```python
from build123d import *

# Parameters (mm, degrees)
SKETCH1_W           = 226
SKETCH1_H           = 170
BOSS_EXTRUDE1_DEPTH = 5
SKETCH2_W           = 226
SKETCH2_H           = 170
BOSS_EXTRUDE2_DEPTH = 4


with BuildPart() as part:
    # Sketch1 → Boss-Extrude1 (new body)
    with BuildSketch(Plane(origin=(0, 0, 0), x_dir=(1, 0, 0), z_dir=(0, 1, 0))):
        Polygon((234, -94), (234, -178), (0, -178), (0, 0), (234, 0), (234, -84), (244, -84), (244, -94), align=None)
        with Locations((117, -89)):
            Rectangle(SKETCH1_W, SKETCH1_H, mode=Mode.SUBTRACT)
    extrude(amount=BOSS_EXTRUDE1_DEPTH)

    # Sketch2 → Boss-Extrude2 (add)
    with BuildSketch(Plane(origin=(0, 0, 0), x_dir=(1, 0, 0), z_dir=(0, 1, 0))):
        with Locations((117, -89)):
            Rectangle(SKETCH2_W, SKETCH2_H)
    extrude(amount=BOSS_EXTRUDE2_DEPTH)


solid = part.part
```
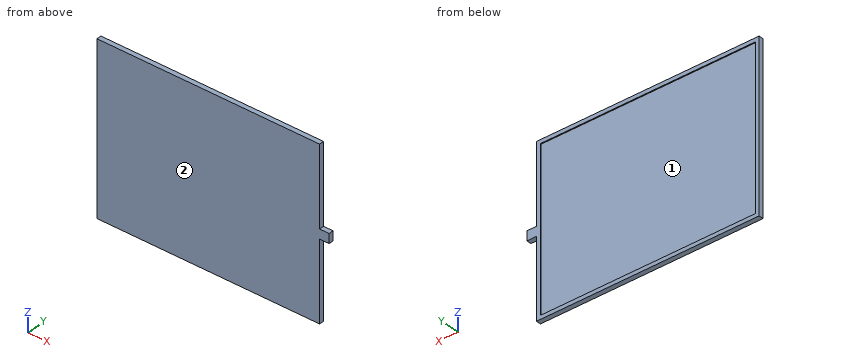
The listing builds one solid part. Answer for the finished solid, in the listing's coordinates (mm). Face numbers are marked on the shaded views. Give positions to 0.01 mm unless a question says otherwise; leave off trailing zeros. Order: outer loops, then holes, each group sorted by start corner. A loop starts at its lowest first (then second) coordinate and runs counter-clockwise, first axis right, second up. Notation, with made-up numbers: (53, 23) -> (62, 23) arc R21 cw to (62, 58) -> close; hole circle Ø5 at (70.5, 36). An arc over 180 degrees is marked (long way). Answer as a JSON object with one key per item and string values. Group by question number.
Item 1: Consider L1, parallel to X at y = 4.5, z = 123.5; L2, parallel to Y at x = 187.5, z = 33.5; L3, parallel to X at y = 3.15, z = 37. Determine where each line is inside the solid, lowest interval first. Write a range as from..to.
Item 2: The part is cut by section B-B on x = 156. Write down the section's boundary in (y, z).
Item 3: The part is cut by section A-A on z = 14.5. Write down the section's boundary in (x, y), and give its area (3 significant figures).
Item 4: Flat-ended cylindrical pins translate along their axes: pin 1 (2.5 mm diameter, centred on y = 1.5, z = 48, fed in from +X); pin 2 (1.5 mm diameter, centred on x = 240, y = 1.5, fed in from -Z). Find the tip coordinate at first contact, or state that the pin passes through.
Item 5: Determine the mould class of the marked faces 1 and 2 for opening direction X: pulls with the +X half, pulls with the -X half, needs draft (parallel to the pull), parting line crosses it, or undercut.
Result set:
{
 "1": {"L1": "0..4, 230..234", "L2": "0..4", "L3": "0..234"},
 "2": {"outline": "(0, 0) -> (5, 0) -> (5, 4) -> (4, 4) -> (4, 174) -> (5, 174) -> (5, 178) -> (0, 178) -> close"},
 "3": {"outline": "(0, 0) -> (234, 0) -> (234, 5) -> (230, 5) -> (230, 4) -> (4, 4) -> (4, 5) -> (0, 5) -> close", "area": "944 mm²"},
 "4": {"pin 1": "x = 234", "pin 2": "z = 84"},
 "5": {"face 1": "undercut", "face 2": "needs draft"}
}
